Could you check a few things on this model? Use its own coordinates, in mm. Coordinates: 2 decimals unless noted, no trailing zeros. Loops run counter-clockwise (first coordinate to the right, second up) from the corner with the lowest first, then second, coordinate; pieces in that order, holes last.
Autodesk Inventor part; units mm, degrees
ref_plane "YZ Plane" through (0, 0, 0) normal (1, 0, 0) x (0, 1, 0)
ref_plane "XZ Plane" through (0, 0, 0) normal (0, 1, 0) x (-1, 0, 0)
ref_plane "XY Plane" through (0, 0, 0) normal (0, 0, 1) x (1, 0, 0)
sketch "Sketch1" plane through (0, 0, 0) normal (0, 1, 0) x (-1, 0, 0)
  circle A0 centre (0, 0) radius 65
  dimension "d0" = 130
extrude "Extrusion1" add sketch "Sketch1" along normal blind 40
sketch "Sketch2" plane through (0, 0, 0) normal (0, -1, 0) x (1, 0, 0)
  line L0 (0, 0) -> (0, 50)
  arc A0 (32.1394, 38.3022) -> (0, 50) centre (0, 0) ccw
  arc A1 (19.2836, 22.9813) -> (0, 30) centre (0, 0) ccw
  line L1 (0, 0) -> (19.2836, 22.9813)
  line L2 (32.1394, 38.3022) -> (19.2836, 22.9813)
  dimension "d4" = 40
  dimension "d5" = 30
  dimension "d6" = 50
extrude "Extrusion2" cut sketch "Sketch2" against normal through all contours L0 A0 L2 A1
pattern_circular "Circular Pattern1" count 6 over 360 about axis through (0, 0, 0) along (0, 1, 0) of "Extrusion2"
properties part number "Large Flywheel"
(1) Imagine slicing it at A-A, the plane z = 0. Write out the boundary of the cut face in (x, y).
Answers:
outline: (-65, 0) - (-50, 0) - (-50, 40) - (-65, 40) - close; (-30, 0) - (30, 0) - (30, 40) - (-30, 40) - close; (50, 0) - (65, 0) - (65, 40) - (50, 40) - close
(2) Imagine slicing it at B-B, the plane y = 14.5. Write out the boundary of the cut face in (x, z), and give its area (3 significant figures).
Answers:
outline: circle Ø130 at (0, 0); hole (-49.24, 8.68) arc R50 ccw to (-43.3, -25) - (-25.98, -15) arc R30 cw to (-29.54, 5.21) - close; hole (-43.3, 25) - (-25.98, 15) arc R30 cw to (-10.26, 28.19) - (-17.1, 46.98) arc R50 ccw to start; hole (-32.14, -38.3) arc R50 ccw to (0, -50) - (0, -30) arc R30 cw to (-19.28, -22.98) - close; hole (0, 30) arc R30 cw to (19.28, 22.98) - (32.14, 38.3) arc R50 ccw to (0, 50) - close; hole (10.26, -28.19) - (17.1, -46.98) arc R50 ccw to (43.3, -25) - (25.98, -15) arc R30 cw to start; hole (25.98, 15) arc R30 cw to (29.54, -5.21) - (49.24, -8.68) arc R50 ccw to (43.3, 25) - close
area: 9,920 mm2
(3) We'd pull the mould along Z, two halves only. Please class faces 1 (the face through (-62, 19.72, -19.52)), 2 (the face through (-13.73, 19.72, 37.72)), 3 (the face through (1, 40, 1)): +Z half, -Z half, draft (parallel to the pull), parting line (faces both ways), or undercut.
Answers:
face 1: parting line
face 2: undercut
face 3: draft
(4) For pin 1 (10 mm diameter, centred on x = -9.5, z = 27.5, fed in from -Y); pin 2 (1 mm diameter, centred on x = -35.5, y = 20.5, fed in from +Z); pin 3 (2 mm diameter, centred on x = 24.5, y = 21.5, fed in from +Z); pin 4 (3 mm diameter, centred on x = 7.5, y = 5.5, fed in from -Z), each with a flat end and sliding along its axis, tell me the tip position at first contact or that it passes through.
Answers:
pin 1: stops at y = 0
pin 2: stops at z = 54.77
pin 3: stops at z = 60.6
pin 4: stops at z = -64.72
(5) I need wall thicknesses on probe 1 along X at (y, z) = (8, -32.5); probe 2 along Z at (x, y) = (20.5, 8); probe 3 along X at (y, z) = (15, 22.5). Which ranges of each line are inside material? Lowest first, please.
Answers:
probe 1: x = -56.29 to -27.27, 0 to 11.83, 38 to 56.29
probe 2: z = -61.68 to -45.6, -21.9 to 24.43, 45.6 to 61.68
probe 3: x = -60.98 to -38.97, -19.84 to 38.97, 44.65 to 60.98
(6) Imagine slicing it at C-C, the plane x = 22. Write out the boundary of the cut face in (y, z).
Answers:
outline: (0, -61.16) - (40, -61.16) - (40, -44.9) - (0, -44.9) - close; (0, -20.4) - (40, -20.4) - (40, 26.22) - (0, 26.22) - close; (0, 44.9) - (40, 44.9) - (40, 61.16) - (0, 61.16) - close
